from build123d import *

# Parameters (mm, degrees)
BOSS_EXTRUDE1_DEPTH = 8
SKETCH3_R           = 1.5
CUT_EXTRUDE1_DEPTH  = 15
SKETCH4_R           = 1.5
CUT_EXTRUDE2_DEPTH  = 10


with BuildPart() as part:
    # Sketch1 → Boss-Extrude1 (new body)
    with BuildSketch(Plane(origin=(0, 0, 0), x_dir=(0, 0, -1), z_dir=(1, 0, 0))):
        with BuildLine():
            Line((17, 0), (20, 0))
            Line((20, 0), (20, -5))
            Line((20, -5), (0, -5))
            Line((0, -5), (0, 0))
            Line((0, 0), (3, 0))
            ThreePointArc((3, 0), (10, 7), (17, 0))
        make_face()
    extrude(amount=BOSS_EXTRUDE1_DEPTH)

    # Sketch3 → Cut-Extrude1 (cut)
    with BuildSketch(Plane.XZ.offset(5)):
        with Locations(Location((3, -5, 0), (0, 0, 270))):
            Circle(SKETCH3_R)
        with Locations(Location((3, -15, 0), (0, 0, 270))):
            Circle(SKETCH3_R)
    extrude(amount=-CUT_EXTRUDE1_DEPTH, mode=Mode.SUBTRACT)

    # Sketch4 → Cut-Extrude2 (cut)
    with BuildSketch(Plane(origin=(8, 0, 0), x_dir=(0, 0, -1), z_dir=(1, 0, 0))):
        with Locations((10, 0)):
            Circle(SKETCH4_R)
    extrude(amount=-CUT_EXTRUDE2_DEPTH, mode=Mode.SUBTRACT)


solid = part.part
Part model, mm, in its own coordinate system. A direction names the side the tool comes from. Give positions to 0.01 mm unless a question says otherwise; leave off trailing zeros. Loops run counter-clockwise (first coordinate to the right, second up) from the corner with the lowest first, then second, coordinate; pieces in that order, holes last.
(1) 3-axis set-ups, long thin cutter, end or side, ignore diameter. For faces 1 (the flat face through (4, 0, -18)), 2 (the flat face through (0, -2, -10)): which of +Z, -Z, +X, -X, +Y, -Y reach the whole face in a straight line?
Return value:
face 1: -Z, +X, -X, +Y
face 2: +Z, -Z, -X, +Y, -Y
(2) Band-saw the part on B-B (z = -10.5). Write the cut outline in (x, y).
Return value:
outline: (0, -5) - (8, -5) - (8, -1.41) - (0, -1.41) - close; (0, 1.41) - (8, 1.41) - (8, 6.98) - (0, 6.98) - close
(3) Band-saw the part on A-A (x = 5.5). Write the cut outline in (y, z).
Return value:
outline: (-5, -20) - (0, -20) - (0, -17) arc R7 ccw to (0, -3) - (0, 0) - (-5, 0) - close; hole circle Ø3 at (0, -10)
(4) Drill centre lines: line 1 along Z through (x, y) = (3, -2); line 2 along Y through (x, z) = (2.5, -10); line 3 along X through (y, z) = (0, -5). Where is each one in solid material? Low to high.
Return value:
line 1: z = -20 to -16.5, -13.5 to -6.5, -3.5 to 0
line 2: y = -5 to -1.5, 1.5 to 7
line 3: x = 0 to 1.5, 4.5 to 8
(5) Pin check, flat tips, straight feed: pin 1 (0.9 mm diameter, centred on x = 5.5, z = -19, fed in from +Y); pin 2 (1.5 mm diameter, centred on x = 7, y = 1.5, fed in from -Z); pin 3 (4 mm diameter, centred on x = 7, y = 3.5, fed in from +Z). Stop position of each tip, or through.
Return value:
pin 1: stops at y = 0
pin 2: stops at z = -16.96
pin 3: stops at z = -3.16
(6) Band-saw the part on C-C (y = -3.25). Write the cut outline in (x, z), and give its area (3 significant figures).
Return value:
outline: (0, -20) - (8, -20) - (8, 0) - (0, 0) - close; hole circle Ø3 at (3, -15); hole circle Ø3 at (3, -5)
area: 146 mm2
(7) Band-saw the part on D-D (x = 3). Write the cut outline in (y, z).
Return value:
outline: (-5, -20) - (0, -20) - (0, -17) arc R7 ccw to (2.6, -16.5) - (-5, -16.5) - close; (-5, -13.5) - (6.06, -13.5) arc R7 ccw to (6.06, -6.5) - (-5, -6.5) - close; (-5, -3.5) - (2.6, -3.5) arc R7 ccw to (0, -3) - (0, 0) - (-5, 0) - close; hole circle Ø3 at (0, -10)
(8) Pull direction Z, two halves, no side cores. Call faces 3 (the cylindrical face through (4, 7, -10)), 4 (the cylindrical face through (3.07, -0.78, -13.5)), 5 (the flat face through (4, 0, -1)): pulls with the +Z half, pulls with the -Z half, needs draft (parallel to the pull), parting line crosses it, or undercut.
Return value:
face 3: parting line crosses it
face 4: undercut
face 5: needs draft
